Autodesk Fusion 360 part; units mm, degrees
sketch "Sketch1" plane through (0, 0, 0) normal (0, 1, 0) x (1, 0, 0)
  line L0 (0, 0) -> (70, 0)
  line L1 (0, 0) -> (0, 60)
  line L2 (70, 0) -> (70, 60)
  circle A0 centre (35, 60) radius 20
  line L3 (60, 15) -> (60, 25)
  line L4 (60, 25) -> (10, 25)
  line L5 (10, 25) -> (10, 15)
  line L6 (10, 15) -> (60, 15)
  arc A1 (70, 60) -> (0, 60) centre (35, 60) ccw
  dimension "d1" = 70
  dimension "d2" = 60
  dimension "d3" = 40
  dimension "d4" = 50
  dimension "d5" = 10
extrude "Extrude1" add sketch "Sketch1" along normal blind 10
Build history of the part. All positions in model axes, mm. A direction names the side the tool comes from. Give positions to 0.01 mm unless a question says otherwise; leave off trailing zeros. Loops run counter-clockwise (first coordinate to the right, second up) from the corner with the lowest first, then second, coordinate; pieces in that order, holes last.
1) Probe line 1 along Z through (x, y) = (35, 5.25); line 2 along X through (y, z) = (6.5, -60); line 3 along Z through (x, y) = (24, 0.5). List the from-to ranges inside material, lowest first.
Values follow:
line 1: z = -95 to -80, -40 to -25, -15 to 0
line 2: x = 0 to 15, 55 to 70
line 3: z = -93.23 to -76.7, -43.3 to -25, -15 to 0
2) Drop flat-ended pins along their axis: P1, Ø6, axis at x = 41.5, y = 3, coming from the +Z side; P2, Ø1.5, axis at x = 7, y = 7, coming from the -Z side. Give the stop position or say it passes through.
Values follow:
P1: stops at z = 0
P2: stops at z = -81.96
3) Two-plate mould, pull along X, no slides. Class faces 3 (the face through (35, 5, 0)), 4 (the face through (35, 5, -15)), 5 (the face through (34.23, 4.93, -94.99)), 6 (the face through (70, 5, -30)): released by +X, released by -X, zero draft, split by the parting line, or undercut.
Values follow:
face 3: zero draft
face 4: undercut
face 5: split by the parting line
face 6: released by +X
4) 3-axis set-ups, long thin cutter, end or side, ignore diameter. For faces 1 (the face through (35, 10, -38)), 2 (the face through (60, 5, -20)): which of +Z, -Z, +X, -X, +Y, -Y reach the whole face in a straight line?
Values follow:
face 1: +Z, -Z, +X, -X, +Y
face 2: +Y, -Y
5) Band-saw the part on C-C on x = 56.5. List the corners of the cut face in (y, z), then the cut area to 3 significant figures.
Values follow:
outline: (0, -87.62) - (10, -87.62) - (10, -25) - (0, -25) - close; (0, -15) - (10, -15) - (10, 0) - (0, 0) - close
area: 776 mm2
6) Band-saw the part on A-A on x = 35. List the corners of the cut face in (y, z).
Values follow:
outline: (0, -95) - (10, -95) - (10, -80) - (0, -80) - close; (0, -40) - (10, -40) - (10, -25) - (0, -25) - close; (0, -15) - (10, -15) - (10, 0) - (0, 0) - close
7) Band-saw the part on D-D on z = -79. List the corners of the cut face in (x, y) (3 decimals), then the cut area to 3 significant figures.
Values follow:
outline: (5.606, 0) - (28.755, 0) - (28.755, 10) - (5.606, 10) - close; (41.245, 0) - (64.394, 0) - (64.394, 10) - (41.245, 10) - close
area: 463 mm2
8) Band-saw the part on B-B on y = 7.5. List the corners of the cut face in (x, z), then the cut area to 3 significant figures.
Values follow:
outline: (0, -60) arc R35 ccw to (70, -60) - (70, 0) - (0, 0) - close; hole (10, -25) - (60, -25) - (60, -15) - (10, -15) - close; hole circle Ø40 at (35, -60)
area: 4,370 mm2
